```python
from build123d import *

# Parameters (mm, degrees)
F0_W     = 930
F0_H     = 1825
F1_DEPTH = 10
F3_DEPTH = 50
F5_D     = 8.5
F7_D     = 8.5
F7_DEPTH = 15


with BuildPart() as f1:
    # F0 (on Front) → F1 (new body)
    with BuildSketch(Plane.XZ):
        Rectangle(F0_W, F0_H)
    extrude(amount=F1_DEPTH)

    # F2 (on face) → F3 (join)
    with BuildSketch(Plane(origin=(0, 0, 0), x_dir=(-1, 0, 0), z_dir=(0, 1, 0))):
        Polygon((465, 912.5), (-465, 912.5), (-465, -912.5), (-455, -912.5), (-455, 902.500026), (455.000026, 902.500026), (455.000026, -912.5), (465, -912.5), align=None)
    extrude(amount=F3_DEPTH)

    # F5 (through all)
    with Locations(Plane.XZ.offset(10)):
        with Locations((385, 66), (385, -66)):
            Hole(F5_D / 2)

    # F7
    with Locations(Plane(origin=(-465, 0, 0), x_dir=(0, -1, 0), z_dir=(-1, 0, 0))):
        with Locations((-20.25, 727.5), (-20.25, 667.5), (-20.25, 1157.5), (-20.25, 1097.5), (-20.25, 30), (-20.25, -30)):
            Hole(F7_D / 2, depth=F7_DEPTH)


solid = f1.part
```
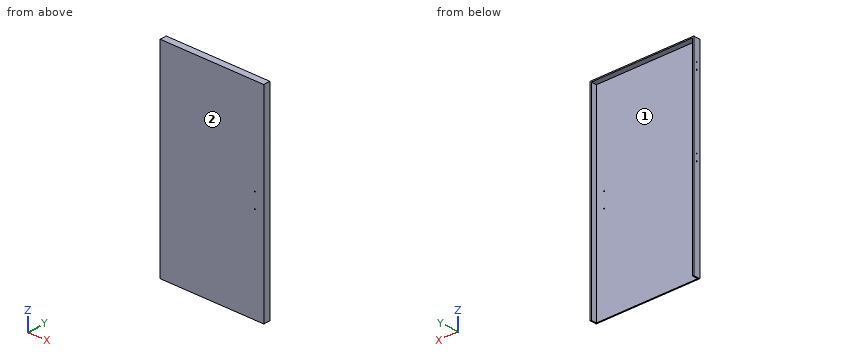
Here's how the part is built. I have some questions about the finished solid (model axes, mm). Face numbers are marked on the shaded views. Coordinates: 2 decimals unless noted, no trailing zeros. Loops run counter-clockwise (first coordinate to the right, second up) from the corner with the lowest first, then second, coordinate; pieces in that order, holes last. Notation, with made-up numbers: (-13, 69) - (36, 69) arc R15 ccw to (36, 86) - close; hole circle Ø6 at (38.5, 43.25). An arc over 180 degrees is marked (long way). Return JSON: item names as keys, results as strings. Group by question number.
Item 1: If we section it at A-A on z = 197: Write out the boundary of the cut face in (x, y).
Item 2: We'd pull the mould along X, two halves only. Please class the marked faces 1 and 2: +X half, -X half, draft (parallel to the pull), parting line (faces both ways), or undercut.
Item 3: If we section it at B-B on x = -143: Write out the boundary of the cut face in (y, z), and give its area (4 significant figures).
Item 4: Will these pins go through, and if not, where does the flat tip stop? P1, Ø7, axis at y = 20.25, z = -30, coming from the -X side; P2, Ø7, axis at x = 385, z = -66, coming from the -Y side; P3, Ø15, axis at x = -80.5, y = 17.5, coming from the -Z side; P4, Ø12, axis at x = -142.5, z = 653.5, coming from the +Y side.
Item 5: I need wall thicknesses on line 1 (Z direction, x = 385, y = -2); line 2 (Z direction, x = -458, y = 20.25); line 3 (X direction, y = 40.5, z = -525.5). Which ranges of each line are inside material? Lowest first, please. Write a range as from..to.
Calculated:
{
 "1": {"outline": "(-465, -10) - (465, -10) - (465, 50) - (455, 50) - (455, 0) - (-455, 0) - (-455, 50) - (-465, 50) - close"},
 "2": {"face 1": "undercut", "face 2": "draft"},
 "3": {"outline": "(-10, -912.5) - (0, -912.5) - (0, 902.5) - (50, 902.5) - (50, 912.5) - (-10, 912.5) - close", "area": "18,750 mm^2"},
 "4": {"P1": "stops at x = 455", "P2": "passes through", "P3": "stops at z = 902.5", "P4": "stops at y = 0"},
 "5": {"line 1": "z = -912.5..-70.25, -61.75..61.75, 70.25..912.5", "line 2": "z = -912.5..-34.25, -25.75..25.75, 34.25..663.25, 671.75..723.25, 731.75..912.5", "line 3": "x = -465..-455, 455..465"}
}
